Could you check a few things on this drawing? It's one solid part, dimensions in mm from its lowest x, y, z. Give positions to 0.01 mm unless a question says otherwise; leave off trailing zeros. Loops run counter-clockwise (first coordinate to the right, second up) from the corner with the lowest first, then second, coordinate; pieces in that order, holes last. Notation, with made-up numbers: (-19, 27) - (34, 27) arc R33 cw to (34, 58) - close; hole circle Ø6 at (87, -26.75). An arc over 180 degrees is marked (long way). Put each result on its own line as item: value. Start each with the question number.
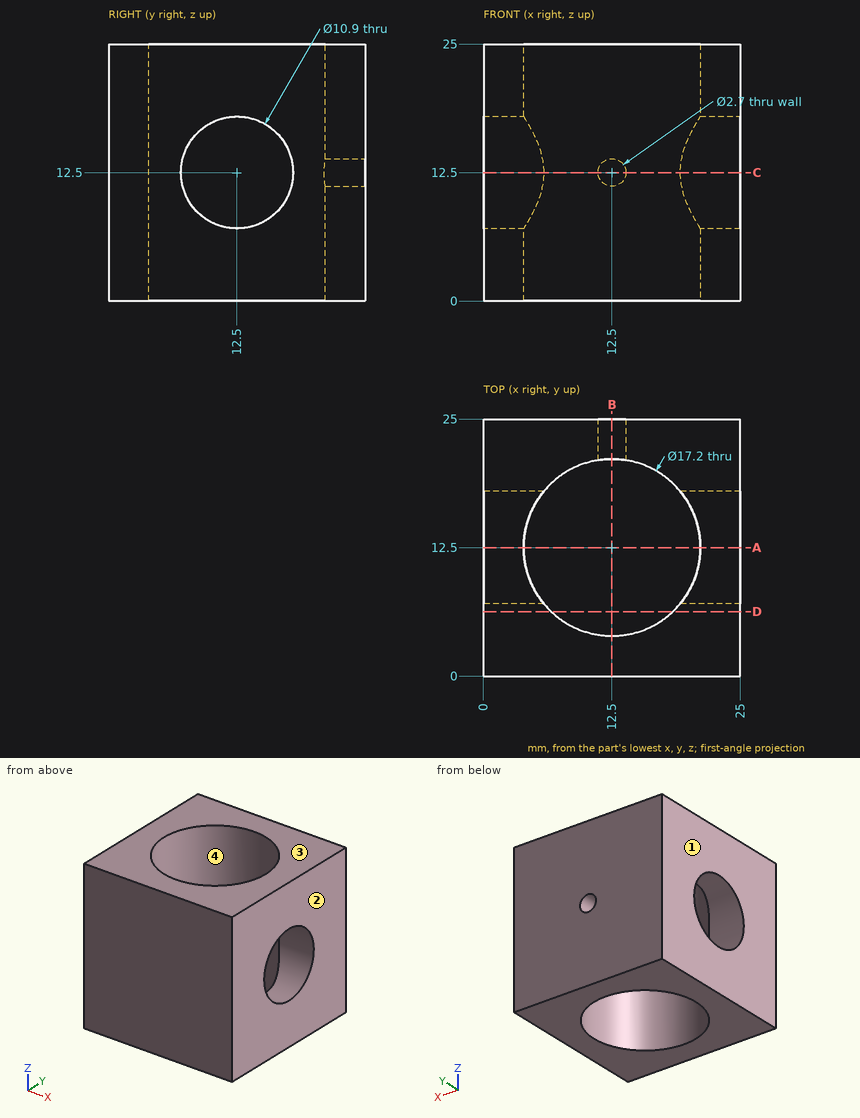
1) Suppose I cut it at C-C on z = 12.5. Please give me the cut outline in (x, y), plus the area to 3 significant figures.
2) Suppose I cut it at D-D on y = 6.25. Please give me the cut outline in (x, z), plus the area to 3 significant figures.
3) Suppose I cut it at B-B on x = 12.5. Please give me the cut outline in (y, z).
4) I need wall thicknesses on line 1 (Z direction, x = 3.85, y = 12.5); line 2 (Z direction, x = 12.5, y = 22); line 3 (Y direction, x = 12.5, z = 11). Which ranges of each line are inside material? Lowest first, please.
5) Suppose I cut it at A-A on y = 12.5. Please give me the cut outline in (x, z).
6) Thinking about a two-plate mould opening in X: for the marked faces 1, 2, 3 and 4, which applies, pulls with the +X half, pulls with the -X half, needs draft (parallel to the pull), parting line crosses it, or undercut?
Ans:
1. outline: (0, 0) - (25, 0) - (25, 7.05) - (19.15, 7.05) arc R8.6 cw to (5.85, 7.05) - (0, 7.05) - close; (0, 17.95) - (5.85, 17.95) arc R8.6 cw to (11.15, 20.99) - (11.15, 25) - (0, 25) - close; (13.85, 20.99) arc R8.6 cw to (19.15, 17.95) - (25, 17.95) - (25, 25) - (13.85, 25) - close
1. area: 284 mm²
2. outline: (0, 0) - (6.59, 0) - (6.59, 25) - (0, 25) - close; (18.41, 0) - (25, 0) - (25, 25) - (18.41, 25) - close
2. area: 330 mm²
3. outline: (0, 0) - (3.9, 0) - (3.9, 25) - (0, 25) - close; (21.1, 0) - (25, 0) - (25, 11.15) - (21.1, 11.15) - close; (21.1, 13.85) - (25, 13.85) - (25, 25) - (21.1, 25) - close
4. line 1: z = 0 to 7.05, 17.95 to 25
4. line 2: z = 0 to 11.15, 13.85 to 25
4. line 3: y = 0 to 3.9, 21.1 to 25
5. outline: (0, 0) - (3.9, 0) - (3.9, 7.05) - (0, 7.05) - close; (0, 17.95) - (3.9, 17.95) - (3.9, 25) - (0, 25) - close; (21.1, 0) - (25, 0) - (25, 7.05) - (21.1, 7.05) - close; (21.1, 17.95) - (25, 17.95) - (25, 25) - (21.1, 25) - close
6. face 1: pulls with the -X half
6. face 2: pulls with the +X half
6. face 3: needs draft
6. face 4: undercut
